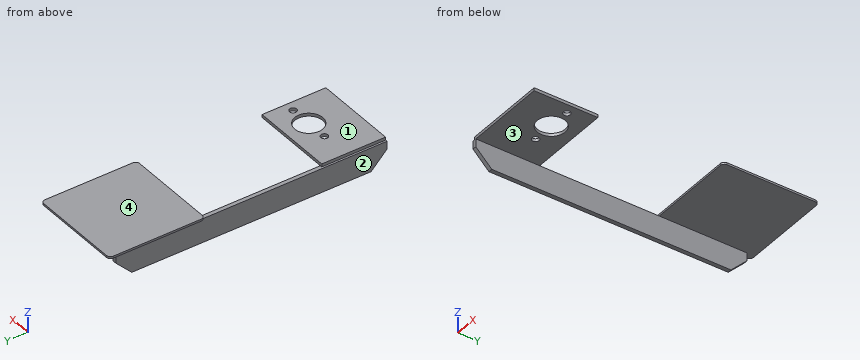
```python
from build123d import *

# Parameters (mm, degrees)
F0_W        = 6.35
F0_H        = 431.8
F1_DEPTH    = 38.1
F2_SIZE     = 25.4
F3_W        = 133.35
F3_H        = 101.6
F4_DEPTH    = 4.7625
F5_R        = 22.225
F5_R_2      = 5.588
F6_DEPTH    = 25.4
F7_W        = 152.4
F7_H        = 152.4
F8_DEPTH    = 3.175
F9_T1_DEPTH = 34.925
F9_T3_DEPTH = 19.05


# Not quite as in the source:
# - a fillet or chamfer that OpenCascade refuses, or shapes differently, is made with other operations: its cross-section is extruded or revolved along the edge and cut away or added


with BuildPart() as f1:
    # F0 (on Top) → F1 (new body)
    with BuildSketch(Plane.XY):
        Rectangle(F0_W, F0_H)
    extrude(amount=-F1_DEPTH)

    # F2
    f2_edges = [f1.edges().sort_by_distance(p)[0] for p in [
        (0, -215.9, -38.1),
        (0, 215.9, -38.1),
    ]]
    chamfer(f2_edges, length=F2_SIZE)

    # F3 (on Top) → F4 (join)
    with BuildSketch(Plane.XY):
        with Locations((66.675, -165.1)):
            Rectangle(F3_W, F3_H)
    extrude(amount=F4_DEPTH)

    # F5 (on face) → F6 (cut)
    with BuildSketch(Plane.XY.offset(4.7625)):
        with Locations((82.55, -152.4)):
            Circle(F5_R)
        with Locations((47.625, -152.4)):
            Circle(F5_R_2)
        with Locations((117.475, -152.4)):
            Circle(F5_R_2)
    extrude(amount=-F6_DEPTH, mode=Mode.SUBTRACT)

    # F7 (on face) → F8 (join)
    with BuildSketch(Plane.XY):
        with Locations((69.85, 152.4)):
            Rectangle(F7_W, F7_H)
    extrude(amount=F8_DEPTH)

    # F9: fillet of radius 6.35 on 4 edges, made by hand

    # F9_s2 → F9_t1 (cut)
    with BuildSketch(Plane.XY.offset(-15.875)):
        with BuildLine():
            ThreePointArc((139.7, 76.2), (144.1901280605, 78.0598719395), (146.05, 82.55))
            Line((146.05, 82.55), (146.05, 76.2))
            Line((146.05, 76.2), (139.7, 76.2))
        make_face()
        with BuildLine():
            ThreePointArc((139.7, 228.6), (144.1901280605, 226.7401280605), (146.05, 222.25))
            Line((146.05, 222.25), (146.05, 228.6))
            Line((146.05, 228.6), (139.7, 228.6))
        make_face()
        with BuildLine():
            ThreePointArc((-6.35, 222.25), (-4.4901280605, 226.7401280605), (0, 228.6))
            Line((0, 228.6), (-6.35, 228.6))
            Line((-6.35, 228.6), (-6.35, 222.25))
        make_face()
    extrude(amount=F9_T1_DEPTH, mode=Mode.SUBTRACT)

    # F9_s4 → F9_t3 (cut)
    with BuildSketch(Plane.XY):
        with BuildLine():
            ThreePointArc((0, 76.2), (-4.4901280605, 78.0598719395), (-6.35, 82.55))
            Line((-6.35, 82.55), (-6.35, 76.2))
            Line((-6.35, 76.2), (0, 76.2))
        make_face()
    extrude(amount=F9_T3_DEPTH, mode=Mode.SUBTRACT)


solid = f1.part
```
Check sheet for the modelled part. Datum: model origin and axes. Units: mm. Face numbers are marked on the shaded views. A direction names the side the tool comes from. Coordinates: 2 decimals unless noted, no trailing zeros. Write each loop counter-clockwise with the first axis right and the second up, starting at its lowest first coordinate (ties: lowest second). Pieces come first, ordered by that corner, then holes. Notation, with made-up numbers: (1.5, 42) -> (18.5, 42) arc R22 cw to (18.5, 56) -> close; hole circle Ø3 at (36.5, 10.25). An arc over 180 degrees is marked (long way). Use a Markdown table: item, result.
1. Sectioned sample at B-B (x = 33). Enter the section's corners in (y, z) (1 decimal), plus the area to 3 significant figures.
Reported:
| item | result |
|---|---|
| outline | (-215.9, 0) -> (-114.3, 0) -> (-114.3, 4.8) -> (-215.9, 4.8) -> close; (76.2, 0) -> (228.6, 0) -> (228.6, 3.2) -> (76.2, 3.2) -> close |
| area | 968 mm2 |
2. Sectioned sample at A-A (y = -152.4). Give the number of separate pieces and of enclosed holes in the cut face, plus the area to 3 significant figures.
Reported:
| item | result |
|---|---|
| separate pieces | 4 |
| enclosed holes | 0 |
| area | 559 mm2 |
3. Sectioned sample at C-C (x = 82.55). Enter the section's corners in (y, z) (1 decimal), plus the area to 3 significant figures.
Reported:
| item | result |
|---|---|
| outline | (-215.9, 0) -> (-174.6, 0) -> (-174.6, 4.8) -> (-215.9, 4.8) -> close; (-130.2, 0) -> (-114.3, 0) -> (-114.3, 4.8) -> (-130.2, 4.8) -> close; (76.2, 0) -> (228.6, 0) -> (228.6, 3.2) -> (76.2, 3.2) -> close |
| area | 756 mm2 |
4. Scan lines: line 1 along Y through (x, z) = (82.55, 1.35) (3 decimals); line 2 along X through (y, z) = (-152, 2); line 3 along Z through (x, y) = (107, 196) (3 decimals). Record each from-to range of solid material in increasing order.
Reported:
| item | result |
|---|---|
| line 1 | y = -215.9 to -174.625, -130.175 to -114.3, 76.2 to 228.6 |
| line 2 | x = 0 to 42.05, 53.2 to 60.33, 104.77 to 111.9, 123.05 to 133.35 |
| line 3 | z = 0 to 3.175 |
5. Tool access check on the marked faces 1, 2, 3 and 4. Record the directions out of +Z, -Z, +X, -X, +Y, -Y that give a thin tool (end or side, any length) a straight path to the whole face; none if there is none.
Reported:
| item | result |
|---|---|
| face 1 | +Z, +X, -X, +Y, -Y |
| face 2 | -Z, -X, +Y, -Y |
| face 3 | -Z, +X, +Y, -Y |
| face 4 | +Z, +X, -X, +Y |
6. Go/stop test with flat-tipped pins: pin 1 Ø6 at (y, z) = (-95.5, -27) entering from +X (3 decimals); pin 2 Ø1.9 at (x, y) = (-1, -110.5) entering from +Z; pin 3 Ø10 at (y, z) = (-62, -5.5) entering from -X (3 decimals); pin 4 Ø18 at (x, y) = (47.625, -152.4) entering from +Z. Record where each tip stops, or that it passes through.
Reported:
| item | result |
|---|---|
| pin 1 | stops at x = 3.175 |
| pin 2 | stops at z = 0 |
| pin 3 | stops at x = -3.175 |
| pin 4 | stops at z = 4.76 |
7. Sectioned sample at D-D (z = -16.5). Enter the section's corners in (x, y) (3 decimals), plus the area to 3 significant figures.
Reported:
| item | result |
|---|---|
| outline | (-3.175, -212.1) -> (3.175, -212.1) -> (3.175, 212.1) -> (-3.175, 212.1) -> close |
| area | 2,690 mm2 |
